Read the model definition and answer for the solid it produces. Units are mm, in the model's axes. A direction names the side the tool comes from. Coordinates: 2 decimals unless noted, no trailing zeros. Order: outer loops, then holes, each group sorted by start corner. A loop starts at its lowest first (then second) coordinate and runs counter-clockwise, first axis right, second up. Notation, with made-up numbers: M 2,-32 L 21,-32 A16 ccw 21,-25 Z; hole C -18,87 d2. An arc over 180 degrees is marked long. One line per question, with ' | ' between items. Start each with the question number.
1) Find section D-D, the plane x = -14. Write down the section's boundary in (y, z).
2) A tool of negligible diameter and unlimited length cuts with its end or side. For faces 1 (the face through (-40, 25, 32)), 2 (the face through (22.594, 29.719, 19.72)), 3 (the face through (42, 25, 16)), from which of +Z, -Z, +X, -X, +Y, -Y can it reach the whole face along a straight path? Write none if from no direction.
3) Find section A-A, the plane y = 12. Write down the section's boundary in (x, z), plus the area to 3 significant figures.
4) The mould has two halves that part along Z. Classify faces 4 (the face through (-1, 36, 40)), 5 (the face through (-14.676, 39.395, 22.146)), 6 (the face through (44.5, 25, 20)): +Z half, -Z half, draft (parallel to the pull), parting line (faces both ways), or undercut.
5) Consider probe 1 along X at (y, z) = (42.25, 20); probe 2 along Y at (x, z) = (32.5, 20); probe 3 along Z at (x, y) = (-14, 38). Determine where each line is inside the solid, lowest interval first.
6) Find section C-C, the plane z = 20. Count the separate pieces of the cut face and the enclosed holes in it, plus the area to 3 significant figures.
7) Given P1, Ø3.5, axis at y = 12, z = 20, coming from the +X side; P2, Ø8, axis at y = 35.5, z = 10.5, coming from the -X side; P3, Ø1.3, axis at x = -42.5, y = 35.5, coming from the +Z side; P4, Ø1, axis at y = 27.5, z = 27.5, coming from the +X side, each flat-ended and moving along its own axis, determine where each tip first touches the part or whether it passes through.
8) Find section B-B, the plane y = 6. Write down the section's boundary in (x, z), plus the area to 3 significant figures.
Autodesk Inventor part; units mm, degrees
ref_plane "YZ Plane" through (0, 0, 0) normal (1, 0, 0) x (0, 1, 0)
ref_plane "XZ Plane" through (0, 0, 0) normal (0, 1, 0) x (-1, 0, 0)
ref_plane "XY Plane" through (0, 0, 0) normal (0, 0, 1) x (1, 0, 0)
sketch "Skizze1" plane through (0, 0, 0) normal (0, 0, 1) x (1, 0, 0)
  line L0 (25, 49) -> (40, 49)
  line L1 (40, 49) -> (40, 0)
  line L2 (40, 0) -> (25, 0)
  line L3 (25, 0) -> (25, 24)
  line L4 (17, 32) -> (0, 32)
  line L5 (0, 32) -> (0, 0) construction
  line L6 (0, -9.8) -> (0, 58.8) construction
  line L7 (-56, 0) -> (56, 0) construction
  line L8 (0, 47) -> (25, 47)
  line L9 (25, 47) -> (25, 49)
  arc A0 (25, 24) -> (17, 32) centre (17, 24) ccw
  line L10 (25, 12) -> (40, 12) construction
  line L11 (-25, 49) -> (-40, 49)
  line L12 (-40, 49) -> (-40, 0)
  line L13 (-40, 0) -> (-25, 0)
  line L14 (-25, 0) -> (-25, 24)
  line L15 (-17, 32) -> (0, 32)
  line L16 (0, 47) -> (-25, 47)
  line L17 (-25, 47) -> (-25, 49)
  arc A1 (-17, 32) -> (-25, 24) centre (-17, 24) ccw
  line L18 (-25, 12) -> (-40, 12) construction
  line L19 (25, 14.5) -> (40, 14.5) construction
  line L20 (40, 14.5) -> (40, 9.5) construction
  line L21 (40, 9.5) -> (25, 9.5) construction
  line L22 (25, 9.5) -> (25, 14.5) construction
  dimension "d0" = 15
  dimension "d1" = 2
  dimension "d2" = 80
  dimension "d4" = 50
  dimension "d5" = 8
  dimension "d6" = 12
  dimension "d7" = 15
  dimension "d8" = 5
extrude "Extrusion1" add sketch "Skizze1" along normal blind 40
sketch "Skizze2" plane through (-25, 47, 0) normal (0, 1, 0) x (1, 0, 0)
  line L0 (50, 0) -> (0, 0) construction
  line L1 (0, 0) -> (0, -40) construction
  line L2 (50, -40) -> (0, -40) construction
  line L3 (50, 0) -> (50, -40) construction
  line L4 (0, 0) -> (0, -40) construction
  line L5 (0, -20) -> (50, -20) construction
  line L6 (50, 0) -> (50, -40) construction
  line L7 (25, -20) -> (25, -40) construction
  line L8 (50, -40) -> (0, -40) construction
  point P0 (25, 0)
  point P1 (11, -20)
  point P2 (39, -20)
  dimension "d11" = 14
  dimension "d12" = 14
hole "Bohrung1" at (-14, 47, 20) at (14, 47, 20) direction (0, -1, 0) diameter 4.5 end through all
sketch "Skizze3" plane through (-40, 0, 0) normal (-1, 0, 0) x (0, 0, 1)
  line L0 (0, 24) -> (0, 0) construction
  line L1 (0, 0) -> (40, 0) construction
  line L2 (40, 24) -> (40, 0) construction
  line L3 (0, 24) -> (40, 24) construction
  line L4 (0, 24) -> (40, 24) construction
  line L5 (20, 24) -> (20, 12) construction
  line L6 (20, 12) -> (40, 12) construction
  point P0 (0, 0)
hole "Bohrung2" at (-40, 12, 20) direction (1, 0, 0) diameter 5.5 end through all
sketch "Skizze4" plane through (40, 0, 0) normal (1, 0, 0) x (0, 0, -1)
  circle A0 centre (-20, 12) radius 2.75 construction
  line L0 (0, 0) -> (0, 49) construction
  line L1 (0, 49) -> (-40, 49) construction
  line L2 (-40, 0) -> (-40, 49) construction
  line L3 (0, 0) -> (-40, 0) construction
  line L4 (0, 0) -> (-40, 0) construction
  line L5 (-20, 0) -> (-20, 49) construction
  line L6 (-24, 49) -> (-16, 49)
  line L7 (-16, 49) -> (-16, 0)
  line L8 (-16, 0) -> (-24, 0)
  line L9 (-24, 0) -> (-24, 49)
  line L10 (-24, 49) -> (-16, 0) construction
  line L11 (-16, 49) -> (-24, 0) construction
  point P0 (-20, 24.5)
  dimension "d28" = 8
extrude "Extrusion2" add sketch "Skizze4" along normal blind 4.5
ref_plane "Arbeitsebene1" through (0, 0, 0) normal (-1, 0, 0) x (0, 0, 1)
mirror "Spiegeln1" about plane through (0, 0, 0) normal (-1, 0, 0) of "Extrusion2"
delete faces "Fläche löschen1" heal yes whole lump no faces at (40, 10.7843, 19.0833)
delete faces "Fläche löschen2" heal yes whole lump no faces at (-40, 12.2194, 20.89)
equation "\"d2\" = Motor_Frame_FixationPlate_Width"
equation "\"d4\" = Fixation_Width"
equation "\"d9\" = Fixation_Thickness"
equation "\"Motor_Frame_FixationPlate_Width\" = 80"
properties part number "Motor_MainAxis_Frame_Fixation" material "PBT-Kunststoff"
Report:
1) outline: M 32,0 L 47,0 L 47,17.75 L 32,17.75 Z; M 32,22.25 L 47,22.25 L 47,40 L 32,40 Z
2) face 1: +Z, -X, +Y, -Y | face 2: +Z, -Z, -Y | face 3: -Z, +X, +Y, -Y
3) outline: M -44.5,16 L -40,16 L -40,0 L -25,0 L -25,17.25 L -44.5,17.25 Z; M -44.5,22.75 L -25,22.75 L -25,40 L -40,40 L -40,24 L -44.5,24 Z; M 25,0 L 40,0 L 40,16 L 44.5,16 L 44.5,17.25 L 25,17.25 Z; M 25,22.75 L 44.5,22.75 L 44.5,24 L 40,24 L 40,40 L 25,40 Z | area: 1,060 mm^2
4) face 4: +Z half | face 5: undercut | face 6: draft
5) probe 1: x = -44.5 to -16.25, -11.75 to 11.75, 16.25 to 44.5 | probe 2: y = 0 to 9.25, 14.75 to 49 | probe 3: z = 0 to 17.75, 22.25 to 40
6) separate pieces: 5 | enclosed holes: 0 | area: 2,340 mm^2
7) P1: passes through | P2: stops at x = -40 | P3: stops at z = 24 | P4: stops at x = 40
8) outline: M -44.5,16 L -40,16 L -40,0 L -25,0 L -25,40 L -40,40 L -40,24 L -44.5,24 Z; M 25,0 L 40,0 L 40,16 L 44.5,16 L 44.5,24 L 40,24 L 40,40 L 25,40 Z | area: 1,270 mm^2
